Could you check a few things on this model? Use its own coordinates, in mm. A direction names the side the tool comes from. Give positions to 0.01 mm unless a question says otherwise; leave off trailing zeros. Write each loop counter-clockwise with the first axis right and the second up, starting at its lowest first coordinate (ties: lowest second). Pieces come first, ordered by that corner, then holes. Notation, with made-up numbers: M 37,62.25 L 51,62.25 A21 cw 51,97.25 Z; hole C -36,-2 d4. An arc over 180 degrees is marked long. Answer as CSV lines item,"result". Start each with the question number.
Autodesk Inventor part; units mm, degrees
ref_plane "YZ Plane" through (0, 0, 0) normal (1, 0, 0) x (0, 1, 0)
ref_plane "XZ Plane" through (0, 0, 0) normal (0, 1, 0) x (-1, 0, 0)
ref_plane "XY Plane" through (0, 0, 0) normal (0, 0, 1) x (1, 0, 0)
sketch "Sketch1" plane through (0, 0, 0) normal (0, 1, 0) x (-1, 0, 0)
  line L0 (0, -31) -> (14, -31)
  line L1 (14, -31) -> (14, 0)
  line L2 (14, 0) -> (7, 0)
  line L3 (0, 0) -> (0, -31)
  line L4 (0.5, -30.5) -> (13.5, -30.5)
  line L5 (13.5, -30.5) -> (13.5, -24.375)
  line L6 (13.5, -24.375) -> (0.5, -24.375)
  line L7 (0.5, -24.375) -> (0.5, -30.5)
  circle A0 centre (7, -7) radius 1.5
  line L8 (7, 0) -> (7, -31) construction
  line L9 (7, 0) -> (0, 0)
  line L10 (13, -14.75) -> (8.25, -14.75)
  line L11 (8.25, -14.75) -> (8.25, -18.75)
  line L12 (8.25, -18.75) -> (13, -18.75)
  line L13 (13, -18.75) -> (13, -14.75)
  dimension "d0" = 14
  dimension "d1" = 31
  dimension "d2" = 0.5
  dimension "d3" = 13
  dimension "d4" = 6.125
  dimension "d5" = 0.5
  dimension "d7" = 3
  dimension "d8" = 7
  dimension "d9" = 1
  dimension "d10" = 14.75
  dimension "d11" = 4
  dimension "d12" = 4.75
extrude "Extrusion1" add sketch "Sketch1" against normal blind 1.3 contours L3 L9 L2 L1 L0 | L7 L6 L5 L4 | L13 L12 L11 L10
extrude "Extrusion2" add sketch "Sketch1" along normal blind 2 contours L7 L6 L5 L4
extrude "Extrusion3" add sketch "Sketch1" along normal blind 1.875 contours L13 L12 L11 L10
sketch "Sketch2" plane through (0, 2, 0) normal (0, 1, 0) x (1, 0, 0)
  line L0 (-13.5, 30.5) -> (-0.5, 30.5)
  line L1 (-0.5, 24.375) -> (-13.5, 24.375)
  line L2 (-4.5, 30.5) -> (-0.5, 30.5)
  line L3 (-0.5, 30.5) -> (-0.5, 24.375)
  line L4 (-0.5, 24.375) -> (-4.5, 24.375)
  line L5 (-4.5, 24.375) -> (-4.5, 30.5)
  line L6 (-13.5, 24.375) -> (-13.5, 30.5)
  line L7 (-13.5, 30.5) -> (-9.5, 30.5)
  line L8 (-9.5, 30.5) -> (-9.5, 24.375)
  line L9 (-9.5, 24.375) -> (-13.5, 24.375)
  line L10 (-13.5, 24.375) -> (-13.5, 30.5)
  point P0 (0, 0)
  dimension "d19" = 4
  dimension "d20" = 4
extrude "Extrusion4" add sketch "Sketch2" along normal blind 8 contours L0 L8 L1 L6 | L0 L3 L1 L5
sketch "Sketch3" plane through (0, 0, 0) normal (1, 0, 0) x (0, 1, 0)
  line L0 (0, 0) -> (0, -31)
  line L1 (0, -3) -> (4.75, -3)
  line L2 (4.75, -3) -> (4.75, -0.5)
  line L3 (4.75, -0.5) -> (0, -0.5)
  line L4 (0, -0.5) -> (0, -3)
  line L5 (0, 0) -> (-1.3, 0)
  line L6 (4.75, -0.5) -> (2.75, -0.5)
  line L7 (2.75, -0.5) -> (2.75, 5.5)
  line L8 (2.75, 5.5) -> (4.75, 5.5)
  line L9 (4.75, 5.5) -> (4.75, -0.5)
  point P0 (0, -0.5)
  dimension "d23" = 4.75
  dimension "d24" = 2.5
  dimension "d25" = 0.5
  dimension "d26" = 8.5
  dimension "d27" = 2
extrude "Extrusion5" add sketch "Sketch3" against normal up to surface (14 mm away)
properties part number "LM393 encoder"
1. Will these pins go through, and if not, where does the flat tip stop? P1, Ø5, axis at y = 6, z = -23, coming from the -X side; P2, Ø3, axis at x = -11, y = 4.5, coming from the -Z side; P3, Ø2.5, axis at x = -5.5, z = 0.5, coming from the +Y side.
2. Imagine slicing it at A-A, the plane y = 7.25. Please give me the cut outline in (x, z) (3 decimals).
3. On a 3-axis mill with a long thin cutter (end or side, diameter ignored), from which of +Z, -Z, +X, -X, +Y, -Y can I reach the whole of each face in a straight line? I mean faces 4 (the flat face through (-4.5, 6, -27)), 5 (the flat face through (-0.5, 5, -27)), 6 (the flat face through (-4, 5, -30.5)), 7 (the flat face through (-4, 5, -24.375)). Say none if no direction works.
4. Imagine slicing it at B-B, the plane y = 3.25. Please give me the cut outline in (x, z) (3 decimals), plus the area to 3 significant figures.
5. Imagine slicing it at D-D, the plane x = -7. Please give me the cut outline in (y, z) (3 decimals), plus the area to 3 significant figures.
6. Thinking about a two-plate mould opening in X: for faces 1 (the flat face through (-11, 1, -14.75)), 2 (the flat face through (-9.5, 6, -27)), 3 (the flat face through (-8.25, 1, -17)), which applies, pulls with the +X half, pulls with the -X half, needs draft (parallel to the pull), parting line crosses it, or undercut?
7. Please list where these lines run through material, in increasing order: line 1 (X direction, y = 7, z = -26); line 2 (Z direction, x = -3, y = 0.75) (3 decimals); line 3 (Z direction, x = -7, y = -0.45).
8. Imagine slicing it at C-C, the plane z = -7. Please give me the cut outline in (x, y), plus the area to 3 significant figures.
Solutions:
1,P1,"x = -13.5"
1,P2,"z = -30.5"
1,P3,"y = 4.75"
2,outline,"M -13.5,-30.5 L -9.5,-30.5 L -9.5,-24.375 L -13.5,-24.375 Z; M -4.5,-30.5 L -0.5,-30.5 L -0.5,-24.375 L -4.5,-24.375 Z"
3,face 4,"-Z, +Y"
3,face 5,"-Z, +X, +Y"
3,face 6,"-Z, +X, -X, +Y"
3,face 7,"+X, -X, +Y"
4,outline,"M -14,-3 L 0,-3 L 0,5.5 L -14,5.5 Z; M -13.5,-30.5 L -9.5,-30.5 L -9.5,-24.375 L -13.5,-24.375 Z; M -4.5,-30.5 L -0.5,-30.5 L -0.5,-24.375 L -4.5,-24.375 Z"
4,area,"168 mm²"
5,outline,"M -1.3,-31 L 0,-31 L 0,-30.5 L 2,-30.5 L 2,-24.375 L 0,-24.375 L 0,-8.5 L -1.3,-8.5 Z; M -1.3,-5.5 L 0,-5.5 L 0,-3 L 4.75,-3 L 4.75,5.5 L 2.75,5.5 L 2.75,-0.5 L 0,-0.5 L 0,0 L -1.3,0 Z"
5,area,"72.5 mm²"
6,face 1,"needs draft"
6,face 2,"undercut"
6,face 3,"pulls with the +X half"
7,line 1,"-13.5 to -9.5, -4.5 to -0.5"
7,line 2,"-30.5 to -24.375, -3 to -0.5"
7,line 3,"-31 to -8.5, -5.5 to 0"
8,outline,"M -14,-1.3 L -8.5,-1.3 L -8.5,0 L -14,0 Z; M -5.5,-1.3 L 0,-1.3 L 0,0 L -5.5,0 Z"
8,area,"14.3 mm²"
